Source: CAD feature listing. Evaluate the final solid. Frame: model axes, mm. A direction names the side the tool comes from. Give positions to 0.01 mm unless a question says otherwise; leave off trailing zeros. Order: outer loops, then holes, each group sorted by start corner. A loop starts at its lowest first (then second) coordinate and runs counter-clockwise, first axis right, second up. Notation, with made-up numbers: (25.25, -32.75) -> (62.25, -32.75) arc R16 ccw to (62.25, -4.75) -> close; hole circle Ø6 at (85.5, 4). An arc over 180 degrees is marked (long way). Use one line per item in the form item = value. Start each with the question number.
from build123d import *

# Parameters (mm, degrees)
SKETCH3_W               = 203.2
SKETCH3_H               = 1.4732
SKETCH4_R               = 2.5527
CUT_EXTRUDE1_DEPTH      = 24.8125
CUT_EXTRUDE1_DEPTH_BACK = 24.8125
CUT_EXTRUDE2_DEPTH      = 24.8125001


with BuildPart() as part:
    # Sketch3 → Revolve1 (revolve)
    with BuildSketch(Plane(origin=(0, 0, 0), x_dir=(0, 0, -1), z_dir=(1, 0, 0))):
        with Locations((0, 23.0759)):
            Rectangle(SKETCH3_W, SKETCH3_H)
    revolve(axis=Axis((0, 0, 101.6), (0, 0, -1)))

    # Sketch4 → Cut-Extrude1 (cut, two sides)
    with BuildSketch(Plane(origin=(0, 0, 0), x_dir=(1, 0, 0), z_dir=(0, 1, 0))) as cut_extrude1_sk:
        with Locations((0, 88.9)):
            Circle(SKETCH4_R)
        with Locations((0, 38.1)):
            Circle(SKETCH4_R)
        with Locations((0, -88.9)):
            Circle(SKETCH4_R)
    extrude(amount=CUT_EXTRUDE1_DEPTH, mode=Mode.SUBTRACT)
    extrude(cut_extrude1_sk.sketch, amount=-CUT_EXTRUDE1_DEPTH_BACK, mode=Mode.SUBTRACT)

    # Sketch5 → Cut-Extrude2 (cut, through all)
    with BuildSketch(Plane(origin=(0, 0, 0), x_dir=(1, 0, 0), z_dir=(0, 1, 0))):
        with BuildLine():
            Line((9.525, -19.05), (-9.525, -19.05))
            ThreePointArc((-9.525, -19.05), (-11.77006403, -18.12006403), (-12.7, -15.875))
            Line((-12.7, -15.875), (-12.7, 15.875))
            ThreePointArc((-12.7, 15.875), (-11.77006403, 18.12006403), (-9.525, 19.05))
            Line((-9.525, 19.05), (9.525, 19.05))
            ThreePointArc((9.525, 19.05), (11.77006403, 18.12006403), (12.7, 15.875))
            Line((12.7, 15.875), (12.7, -15.875))
            ThreePointArc((12.7, -15.875), (11.77006403, -18.12006403), (9.525, -19.05))
        make_face()
    extrude(amount=-CUT_EXTRUDE2_DEPTH, mode=Mode.SUBTRACT)


solid = part.part
1) Cut plane D-D, the plane z = 9.5. Return the cut outline in (x, y) (1 decimal).
2) Cut plane A-A, the plane z = 88.9. Return the cut outline in (x, y) (1 decimal).
3) Draft query along Z for faces 1 (the face through (-18, -14, -101.6)), 2 (the face through (-18, -14, 101.6)), 3 (the face through (0, -23, 19.05)). Return one class per face: +Z half, -Z half, draft (parallel to the pull), parting line (faces both ways), or undercut.
4) Pin query (flat end, axial travel): pin 1 (10 mm diameter, centred on x = 17.5, z = 80, fed in from -Y); pin 2 (1.5 mm diameter, centred on y = 14.5, z = -37, fed in from +X); pin 3 (1.4 mm diameter, centred on y = -19, z = -1, fed in from -X); pin 4 (3 mm diameter, centred on x = 0, z = -38.1, fed in from -Y). Return the tip coordinate at first contact, or that it passes through.
5) Cut plane C-C, the plane x = 0. Count the separate pieces of the cut face and the enclosed holes in it, plus the area to 3 significant figures.
6) Reachability of faces 4 (the face through (0, -23, -19.05)), 5 (the face through (-2.55, -22.99, -38.21)) from +Z, -Z, +X, -X, +Y, -Y: full face, straight path, thin tool, end or side. Return the list, or none.
7) Cut plane B-B, the plane y = 19.5. Return the cut outline in (x, z).
8) Material intervals for probe 1 along Z at (x, y) = (0, 23.1); probe 2 along X at (y, z) = (4, 89); probe 3 along X at (y, z) = (3.5, 56), sorted ascending.
Output values:
q1.outline = (-12.7, -20.1) -> (-12.7, -18.4) arc R22.3 cw (long way) to (12.7, -18.4) -> (12.7, -20.1) arc R23.8 ccw (long way) to start
q2.outline = (-2.6, -23.7) -> (-2.6, -22.2) arc R22.3 cw to (-2.6, 22.2) -> (-2.6, 23.7) arc R23.8 ccw to start; (2.6, -23.7) arc R23.8 ccw to (2.6, 23.7) -> (2.6, 22.2) arc R22.3 cw to (2.6, -22.2) -> close
q3.face_1 = -Z half
q3.face_2 = +Z half
q3.face_3 = undercut
q4.pin_1 = -20.27
q4.pin_2 = 19.44
q4.pin_3 = -15.24
q4.pin_4 = through
q5.separate_pieces = 9
q5.enclosed_holes = 0
q5.area = 497 mm^2
q6.face_4 = -Y
q6.face_5 = +Y, -Y
q7.outline = (-13.67, -101.6) -> (-10.9, -101.6) -> (-10.9, 101.6) -> (-13.67, 101.6) -> close; (10.9, -101.6) -> (13.67, -101.6) -> (13.67, 101.6) -> (10.9, 101.6) -> close
q8.probe_1 = -101.6 to -91.45, -86.35 to -40.65, -35.55 to 86.35, 91.45 to 101.6
q8.probe_2 = -23.47 to -21.98, 21.98 to 23.47
q8.probe_3 = -23.55 to -22.06, 22.06 to 23.55
